The listing builds one solid part. Answer for the finished solid, in the listing's coordinates (mm). Face numbers are marked on the shaded views. Coordinates: 2 decimals unless noted, no trailing zeros. Order: outer loops, then holes, each group sorted by start corner. A loop starts at its lowest first (then second) coordinate and runs counter-clockwise, first axis right, second up. Notation, with made-up numbers: (-14, 71.25) -> (17, 71.25) arc R26 ccw to (17, 101.25) -> close; hole circle Ø7 at (-29, 53). An arc over 180 degrees is marked (long way). Return JSON: item names as keys, results as strings.
```python
from build123d import *

# Parameters (mm, degrees)
SKETCH_1_R             = 1.15
SKETCH_1_R_2           = 15
SKETCH_1_R_3           = 1.25
EXTRUDE_1_DEPTH        = 4
HOLE_WIZARD_M3_1_D     = 2.5
HOLE_WIZARD_M3_1_DEPTH = 7.5
HOLE_WIZARD_M3_1_TIP   = 0.751075774
SKETCH1_R              = 1.25
BOSS_EXTRUDE1_DEPTH    = 0.01
SKETCH1_2_R            = 1.25
BOSS_EXTRUDE2_DEPTH    = 0.01


with BuildPart() as part:
    # 草图1 → 凸台-拉伸1 (new, symmetric)
    with BuildSketch(Plane(origin=(0, 0, 0), x_dir=(0, 0, -1), z_dir=(1, 0, 0))):
        with BuildLine():
            Line((30, -40), (30, 0))
            ThreePointArc((30, 0), (23.323275812, 18.868619595), (6.265012972, 29.3385346))
            ThreePointArc((6.265012972, 29.3385346), (4.402143602, 30.598161767), (3.938008154, 32.798507463))
            ThreePointArc((3.938008154, 32.798507463), (0, 37.5), (-3.938008154, 32.798507463))
            ThreePointArc((-3.938008154, 32.798507463), (-4.402143602, 30.598161767), (-6.265012972, 29.3385346))
            ThreePointArc((-6.265012972, 29.3385346), (-23.323275812, 18.868619595), (-30, 0))
            Line((-30, 0), (-30, -40))
            Line((-30, -40), (30, -40))
        make_face()
        with BuildLine():
            ThreePointArc((4.333333333, 19.012422839), (0, 19.5), (-4.333333333, 19.012422839))
            ThreePointArc((-4.333333333, 19.012422839), (-7.924988129, 21.270744302), (-5.666666667, 24.862399098))
            ThreePointArc((-5.666666667, 24.862399098), (0, 25.5), (5.666666667, 24.862399098))
            ThreePointArc((5.666666667, 24.862399098), (7.924988129, 21.270744302), (4.333333333, 19.012422839))
        make_face(mode=Mode.SUBTRACT)
        with BuildLine():
            ThreePointArc((-5.666666667, -24.862399098), (-7.924988129, -21.270744302), (-4.333333333, -19.012422839))
            ThreePointArc((-4.333333333, -19.012422839), (0, -19.5), (4.333333333, -19.012422839))
            ThreePointArc((4.333333333, -19.012422839), (7.924988129, -21.270744302), (5.666666667, -24.862399098))
            ThreePointArc((5.666666667, -24.862399098), (0, -25.5), (-5.666666667, -24.862399098))
        make_face(mode=Mode.SUBTRACT)
        with Locations((-23.815698604, -13.75)):
            Circle(SKETCH_1_R, mode=Mode.SUBTRACT)
        with BuildLine():
            ThreePointArc((-24.364802551, -7.523722261), (-22.383498987, -3.772131106), (-18.631907833, -5.75343467))
            ThreePointArc((-18.631907833, -5.75343467), (-16.887495374, -9.75), (-14.2985745, -13.258988169))
            ThreePointArc((-14.2985745, -13.258988169), (-14.458510858, -17.498613195), (-18.698135884, -17.338676837))
            ThreePointArc((-18.698135884, -17.338676837), (-22.083647797, -12.75), (-24.364802551, -7.523722261))
        make_face(mode=Mode.SUBTRACT)
        with Locations((-15.155444566, -8.75)):
            Circle(SKETCH_1_R, mode=Mode.SUBTRACT)
        with Locations((0, -27.5)):
            Circle(SKETCH_1_R, mode=Mode.SUBTRACT)
        with Locations((0, -17.5)):
            Circle(SKETCH_1_R, mode=Mode.SUBTRACT)
        with BuildLine():
            ThreePointArc((18.631907833, -5.75343467), (22.383498987, -3.772131106), (24.364802551, -7.523722261))
            ThreePointArc((24.364802551, -7.523722261), (22.083647797, -12.75), (18.698135884, -17.338676837))
            ThreePointArc((18.698135884, -17.338676837), (14.458510858, -17.498613195), (14.2985745, -13.258988169))
            ThreePointArc((14.2985745, -13.258988169), (16.887495374, -9.75), (18.631907833, -5.75343467))
        make_face(mode=Mode.SUBTRACT)
        with Locations((23.815698604, -13.75)):
            Circle(SKETCH_1_R, mode=Mode.SUBTRACT)
        with Locations((15.155444566, -8.75)):
            Circle(SKETCH_1_R, mode=Mode.SUBTRACT)
        with Locations((-23.815698604, 13.75)):
            Circle(SKETCH_1_R, mode=Mode.SUBTRACT)
        with BuildLine():
            ThreePointArc((-18.698135884, 17.338676837), (-14.458510858, 17.498613195), (-14.2985745, 13.258988169))
            ThreePointArc((-14.2985745, 13.258988169), (-16.887495374, 9.75), (-18.631907833, 5.75343467))
            ThreePointArc((-18.631907833, 5.75343467), (-22.383498987, 3.772131106), (-24.364802551, 7.523722261))
            ThreePointArc((-24.364802551, 7.523722261), (-22.083647797, 12.75), (-18.698135884, 17.338676837))
        make_face(mode=Mode.SUBTRACT)
        with Locations((-15.155444566, 8.75)):
            Circle(SKETCH_1_R, mode=Mode.SUBTRACT)
        Circle(SKETCH_1_R_2, mode=Mode.SUBTRACT)
        with Locations((0, 17.5)):
            Circle(SKETCH_1_R, mode=Mode.SUBTRACT)
        with Locations((0, 27.5)):
            Circle(SKETCH_1_R, mode=Mode.SUBTRACT)
        with Locations((0, 33.5)):
            Circle(SKETCH_1_R_3, mode=Mode.SUBTRACT)
        with Locations((15.155444566, 8.75)):
            Circle(SKETCH_1_R, mode=Mode.SUBTRACT)
        with BuildLine():
            ThreePointArc((24.364802551, 7.523722261), (22.383498987, 3.772131106), (18.631907833, 5.75343467))
            ThreePointArc((18.631907833, 5.75343467), (16.887495374, 9.75), (14.2985745, 13.258988169))
            ThreePointArc((14.2985745, 13.258988169), (14.458510858, 17.498613195), (18.698135884, 17.338676837))
            ThreePointArc((18.698135884, 17.338676837), (22.083647797, 12.75), (24.364802551, 7.523722261))
        make_face(mode=Mode.SUBTRACT)
        with Locations((23.815698604, 13.75)):
            Circle(SKETCH_1_R, mode=Mode.SUBTRACT)
    extrude(amount=EXTRUDE_1_DEPTH, both=True)

    # M3 螺纹孔1
    with Locations(Plane(origin=(0, -40, 22.5), x_dir=(0, 0, -1), z_dir=(0, -1, 0))):
        with Locations((0, 0), (22.5, 0), (45, 0)):
            Hole(HOLE_WIZARD_M3_1_D / 2, depth=HOLE_WIZARD_M3_1_DEPTH)
            with Locations((0, 0, -(HOLE_WIZARD_M3_1_DEPTH + HOLE_WIZARD_M3_1_TIP / 2))):  # 118° drill point
                Cone(0, HOLE_WIZARD_M3_1_D / 2, HOLE_WIZARD_M3_1_TIP, mode=Mode.SUBTRACT)

    # Sketch1 → Boss-Extrude1 (add)
    with BuildSketch(Plane(origin=(4, 0, 0), x_dir=(0, 0, -1), z_dir=(1, 0, 0))):
        with BuildLine():
            Line((-3.938008154, 32.798507463), (-3.526843322, 30.490328295))
            Line((-3.526843322, 30.490328295), (3.526843322, 30.490328295))
            Line((3.526843322, 30.490328295), (3.938008154, 32.798507463))
            ThreePointArc((3.938008154, 32.798507463), (0, 37.5), (-3.938008154, 32.798507463))
        make_face()
        with Locations((0, 33.5)):
            Circle(SKETCH1_R, mode=Mode.SUBTRACT)
    extrude(amount=BOSS_EXTRUDE1_DEPTH)

    # Sketch1<2> → Boss-Extrude2 (add)
    with BuildSketch(Plane(origin=(4, 0, 0), x_dir=(0, 0, -1), z_dir=(1, 0, 0))):
        with BuildLine():
            Line((-3.938008154, 32.798507463), (-3.526843322, 30.490328295))
            Line((-3.526843322, 30.490328295), (3.526843322, 30.490328295))
            Line((3.526843322, 30.490328295), (3.938008154, 32.798507463))
            ThreePointArc((3.938008154, 32.798507463), (0, 37.5), (-3.938008154, 32.798507463))
        make_face()
        with Locations((0, 33.5)):
            Circle(SKETCH1_2_R, mode=Mode.SUBTRACT)
    extrude(amount=BOSS_EXTRUDE2_DEPTH)


solid = part.part
```
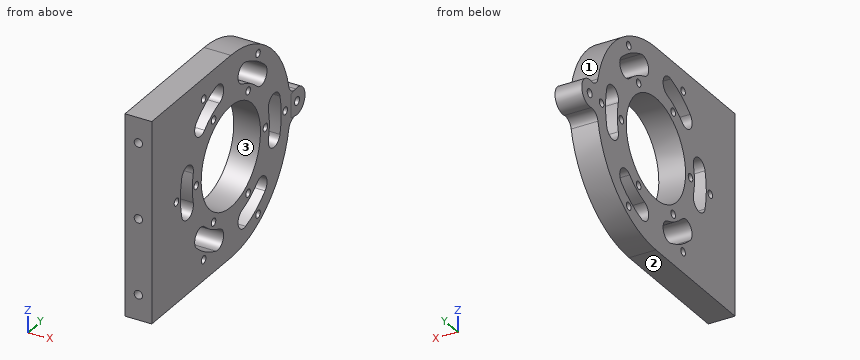
Item 1: Flat-ended cylindrical pins translate along their axes: pin 1 (1.8 mm diameter, centred on y = 13.75, z = 23.82, fed in from +X); pin 2 (4 mm diameter, centred on x = 0, z = -22.5, fed in from +Y); pin 3 (10 mm diameter, centred on y = 29, z = 14, fed in from +X); pin 4 (3 mm diameter, centred on x = -0.5, z = 11.5, fed in from +Y). Find the tip coordinate at first contact, or state that the pin passes through.
Answer list:
{"pin 1": "through", "pin 2": "y = 21.9", "pin 3": "x = 4", "pin 4": "y = 28.28"}
Item 2: Determine the mould class of the marked faces 1, 2 and 3 for opening direction Z: pulls with the +Z half, pulls with the -Z half, needs draft (parallel to the pull), parting line crosses it, or undercut.
Answer list:
{"face 1": "pulls with the +Z half", "face 2": "pulls with the -Z half", "face 3": "undercut"}
Item 3: The part is cut by section B-B on y = 21. Determine the outline of the cut face in (x, z), plus the area to 3 significant figures.
Answer list:
{"outline": "(-4, -21.42) -> (4, -21.42) -> (4, -7.85) -> (-4, -7.85) -> close; (-4, 7.85) -> (4, 7.85) -> (4, 21.42) -> (-4, 21.42) -> close", "area": "217 mm2"}
Item 4: The part is cut by section D-D on y = 8.75. Determine the outline of the cut face in (x, z), plus the area to 3 significant figures.
Answer list:
{"outline": "(-4, -28.7) -> (4, -28.7) -> (4, -23.95) -> (-4, -23.95) -> close; (-4, -17.43) -> (4, -17.43) -> (4, -16.31) -> (-4, -16.31) -> close; (-4, -14.01) -> (4, -14.01) -> (4, -12.18) -> (-4, -12.18) -> close; (-4, 12.18) -> (4, 12.18) -> (4, 14.01) -> (-4, 14.01) -> close; (-4, 16.31) -> (4, 16.31) -> (4, 17.43) -> (-4, 17.43) -> close; (-4, 23.95) -> (4, 23.95) -> (4, 28.7) -> (-4, 28.7) -> close", "area": "123 mm2"}
Item 5: The part is cut by section A-A on z = 11. Determine the outline of the cut face in (x, y).
Answer list:
{"outline": "(-4, -40) -> (4, -40) -> (4, -10.2) -> (-4, -10.2) -> close; (-4, 10.2) -> (4, 10.2) -> (4, 27.91) -> (-4, 27.91) -> close"}
Item 6: The part is cut by section C-C on z = -20. Determine the outline of the cut face in (x, y).
Answer list:
{"outline": "(-4, -40) -> (4, -40) -> (4, -15.82) -> (-4, -15.82) -> close; (-4, -4.04) -> (4, -4.04) -> (4, 4.04) -> (-4, 4.04) -> close; (-4, 15.82) -> (4, 15.82) -> (4, 22.36) -> (-4, 22.36) -> close"}
Item 7: Find the intervals of material crossed by probe 1 along Y at (x, z) = (2.75, -6); probe 2 along Y at (x, z) = (-3, -18); probe 3 along Z at (x, y) = (-1.5, -15.5), in increasing order.
Answer list:
{"probe 1": "-40 to -24.77, -19.11 to -13.75, 13.75 to 19.11, 24.77 to 29.41", "probe 2": "-40 to -17.9, -7.5 to 7.5, 17.9 to 24", "probe 3": "-30 to -20.25, -13.51 to 13.51, 20.25 to 30"}
